The drawing under review shows one solid part. Ordinate dimensions are in mm from its lowest x, y, z. Coordinates: 2 decimals unless noted, no trailing zeros. Loops run counter-clockwise (first coordinate to the right, second up) from the corner with the lowest first, then second, coordinate; pieces in that order, holes last. Notation, with made-up numbers: M 74,63.5 L 94,63.5 A16 cw 94,93.5 Z; hole C -5.5,-15.5 d4. An arc over 180 degrees is marked long. Answer as a JSON object with one key per item and string values. Group by question number.
1. Insertion check: pin 1 (0.9 mm diameter, centred on y = 20.5, z = 2, fed in from -X); pin 2 (1.5 mm diameter, centred on x = 19, z = 1.5, fed in from -Y); pin 3 (0.9 mm diameter, centred on x = 21, z = 1, fed in from +Y). Each pin has a flat end and moves straight along its axis. Give the tip position at first contact, or say it passes through.
2. Consider section A-A (y = 60). State the section outline as (x, z) points.
3. To check wall thickness, follow probe 1 along Y at (x, z) = (60, 1.75); probe 2 along X at (y, z) = (84.5, 1.9); probe 3 along Y at (x, z) = (35, 2) (1 decimal). State the ranges of each line that lie inside material, in increasing order.
4. Consider section C-C (z = 2.15). Count the separate pieces of the cut face and the enclosed holes in it, then the cut area to 3 significant figures.
5. Consider section D-D (x = 17.5). State the section outline as (y, z) points.
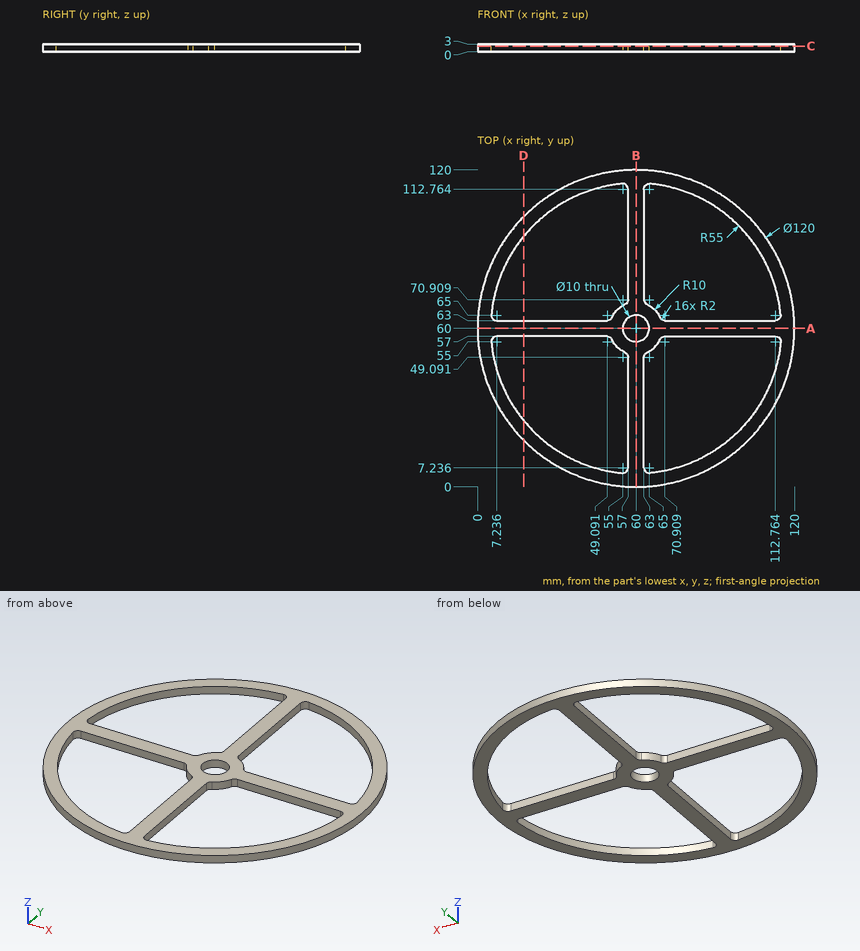
Findings below:
{
 "1": {"pin 1": "stops at x = 14.45", "pin 2": "stops at y = 15.5", "pin 3": "stops at y = 105.98"},
 "2": {"outline": "M 0,0 L 55,0 L 55,3 L 0,3 Z; M 65,0 L 120,0 L 120,3 L 65,3 Z"},
 "3": {"probe 1": "y = 0 to 55, 65 to 120", "probe 2": "x = 5.23 to 10.76, 57 to 63, 109.24 to 114.77", "probe 3": "y = 5.5 to 11, 57 to 63, 109 to 114.5"},
 "4": {"separate pieces": "1", "enclosed holes": "5", "area": "3,140 mm^2"},
 "5": {"outline": "M 17.65,0 L 25.09,0 L 25.09,3 L 17.65,3 Z; M 57,0 L 63,0 L 63,3 L 57,3 Z; M 94.91,0 L 102.35,0 L 102.35,3 L 94.91,3 Z"}
}
